Work out the finished part from the listing and answer in its coordinate system (mm). A direction names the side the tool comes from. Round coordinates to 2 decimals unless told otherwise and drop trailing zeros. Loops run counter-clockwise (first coordinate to the right, second up) from the corner with the lowest first, then second, coordinate; pieces in that order, holes last.
```python
from build123d import *

# Parameters (mm, degrees)
BOSS_EXTRUDE1_DEPTH = 16
CUT_EXTRUDE2_DEPTH  = 16
BOSS_EXTRUDE2_DEPTH = 12
FILLET3_R           = 2


with BuildPart() as part:
    # Sketch4 → Boss-Extrude1 (new body)
    with BuildSketch(Plane(origin=(0, 0, 0), x_dir=(1, 0, 0), z_dir=(0, 1, 0))):
        with BuildLine():
            Line((-59, -22), (37, -22))
            ThreePointArc((37, -22), (59, 0), (37, 22))
            Line((37, 22), (-59, 22))
            Line((-59, 22), (-59, -22))
        make_face()
    extrude(amount=BOSS_EXTRUDE1_DEPTH)

    # Sketch6 → Cut-Extrude2 (cut)
    with BuildSketch(Plane(origin=(0, 16, 0), x_dir=(1, 0, 0), z_dir=(0, 1, 0))):
        with BuildLine():
            Line((37, -8), (13, -8))
            ThreePointArc((13, -8), (5, 0), (13, 8))
            Line((13, 8), (37, 8))
            ThreePointArc((37, 8), (45, 0), (37, -8))
        make_face()
    extrude(amount=-CUT_EXTRUDE2_DEPTH, mode=Mode.SUBTRACT)

    # Sketch9 → Boss-Extrude2 (add)
    with BuildSketch(Plane(origin=(0, 0, -22), x_dir=(-1, 0, 0), z_dir=(0, 0, -1))):
        with BuildLine():
            Line((11, 16), (59, 16))
            Line((59, 16), (59, 56))
            ThreePointArc((59, 56), (35, 32), (11, 56))
            Line((11, 56), (11, 16))
        make_face()
        with BuildLine():
            ThreePointArc((11, 56), (35, 32), (59, 56))
            Line((59, 56), (45.408831702, 56))
            ThreePointArc((45.408831702, 56), (35, 45.591168298), (24.591168298, 56))
            Line((24.591168298, 56), (11, 56))
        make_face()
        with BuildLine():
            Line((45.408831702, 56), (59, 56))
            ThreePointArc((59, 56), (35, 80), (11, 56))
            Line((11, 56), (24.591168298, 56))
            ThreePointArc((24.591168298, 56), (35, 66.408831702), (45.408831702, 56))
        make_face()
    boss_extrude2 = extrude(amount=-BOSS_EXTRUDE2_DEPTH)

    # Mirror5: Boss-Extrude2 across plane
    add(boss_extrude2.mirror(Plane.XY))

    # Fillet3
    fillet3_edges = [part.edges().sort_by_distance(p)[0] for p in [
        (-11, 16, -16),
        (-35, 16, -10),
        (-35, 16, 10),
        (-11, 16, 16),
    ]]
    fillet(fillet3_edges, radius=FILLET3_R)


solid = part.part
```
1. Given pin 1 (12 mm diameter, centred on x = -3, z = -11.5, fed in from +Y); pin 2 (18.5 mm diameter, centred on x = -35, y = 56, fed in from +Z); pin 3 (13 mm diameter, centred on y = 45.5, z = -14, fed in from +X); pin 4 (3 mm diameter, centred on x = -26, z = 10, fed in from +Y), each flat-ended and moving along its own axis, determine where each tip first touches the part or whether it passes through.
Answer key:
pin 1: stops at y = 16
pin 2: passes through
pin 3: stops at x = -11
pin 4: stops at y = 78.8
2. Consider probe 1 along Y at (x, z) = (-35, -13); probe 2 along Z at (x, y) = (-38.5, 46); probe 3 along X at (y, z) = (6.5, -2). Determine where each line is inside the solid, lowest interval first.
Answer key:
probe 1: y = 0 to 45.59, 66.41 to 80
probe 2: z = -22 to -10, 10 to 22
probe 3: x = -59 to 5.25, 44.75 to 58.91
3. Find section A-A (z = 0). Write down the section's boundary in (x, y), then the cut area to 3 significant figures.
Answer key:
outline: (-59, 0) - (5, 0) - (5, 16) - (-59, 16) - close; (45, 0) - (59, 0) - (59, 16) - (45, 16) - close
area: 1,250 mm2
4. Find section C-C (y = 5.5). Write down the section's boundary in (x, z), then the cut area to 3 significant figures.
Answer key:
outline: (-59, -22) - (37, -22) arc R22 ccw to (37, 22) - (-59, 22) - close; hole (13, -8) - (37, -8) arc R8 ccw to (37, 8) - (13, 8) arc R8 ccw to start
area: 4,400 mm2
5. Find section B-B (x = 18.5). Write down the section's boundary in (y, z).
Answer key:
outline: (0, -22) - (16, -22) - (16, -8) - (0, -8) - close; (0, 8) - (16, 8) - (16, 22) - (0, 22) - close
6. Find section D-D (x = -35). Write down the section's boundary in (y, z).
Answer key:
outline: (0, -22) - (45.59, -22) - (45.59, -10) - (18, -10) arc R2 cw to (16, -8) - (16, 8) arc R2 cw to (18, 10) - (45.59, 10) - (45.59, 22) - (0, 22) - close; (66.41, -22) - (80, -22) - (80, -10) - (66.41, -10) - close; (66.41, 10) - (80, 10) - (80, 22) - (66.41, 22) - close
7. Determine the mould class of faces 4 (the face through (-35, 43, 10)), 5 (the face through (-59, 15, 0)), 6 (the face through (25, 8, 8)), 7 (the face through (-11, 37, -16)) for opening direction X: +X half, -X half, draft (parallel to the pull), parting line (faces both ways), or undercut.
Answer key:
face 4: draft
face 5: -X half
face 6: undercut
face 7: +X half
8. Which of the six approach directions +Z, -Z, +X, -X, +Y, -Y give full straight-line access (tool end or side, diameter ignored) to faces 1 (the face through (-11, 37, 16)), 2 (the face through (25, 8, -8)), 3 (the face through (-35, 43, -10))?
Answer key:
face 1: +Z, -Z, +X, +Y
face 2: +Y, -Y
face 3: +X, -X, +Y
